Input: part model. Units: mm. Frame: model coordinates. Round coordinates to 2 decimals unless told otherwise and drop trailing zeros. Order: outer loops, then holes, each group sorted by start corner. A loop starts at its lowest first (then second) coordinate and runs counter-clockwise, first axis right, second up. Notation, with made-up numbers: (-17, -28.75) -> (19, -28.75) arc R27 cw to (19, -10.75) -> close; hole circle Ø6 at (39, 28.5). An arc over 180 degrees is marked (long way). Use a Markdown table: item, result.
from build123d import *

# Parameters (mm, degrees)
BASE_DEPTH               = 5
ESQUISSE8_R              = 5
ENL_V_MAT_EXTRU_7_DEPTH  = 10
ESQUISSE4_R              = 11
ESQUISSE4_R_2            = 3.5
ESQUISSE4_RX             = 1.5
ESQUISSE4_RY             = 0.5
ESQUISSE4_W              = 20
ESQUISSE4_H              = 14
ENL_V_MAT_EXTRU_8_DEPTH  = 10
ESQUISSE2_R              = 3
ESQUISSE2_R_2            = 2.5
ENL_V_MAT_EXTRU_9_DEPTH  = 10
ESQUISSE11_R             = 1.5
ENL_V_MAT_EXTRU_11_DEPTH = 5


with BuildPart() as part:
    # Esquisse1 → Base (new body)
    with BuildSketch(Plane.XY):
        Polygon((0, 0), (-175, 0), (-199.748737342, 24.748737342), (-199.748737342, 284.748737342), (-175, 309.497474683), (0, 309.497474683), (24.748737342, 284.748737342), (24.748737342, 24.748737342), align=None)
    extrude(amount=BASE_DEPTH)

    # Esquisse8 → Enlèv. mat.-Extru.7 (cut)
    with BuildSketch(Plane.XY.offset(5)):
        with Locations((-120.5, 286.497474683)):
            Circle(ESQUISSE8_R)
    extrude(amount=-ENL_V_MAT_EXTRU_7_DEPTH, mode=Mode.SUBTRACT)

    # Esquisse4 → Enlèv. mat.-Extru.8 (cut)
    with BuildSketch(Plane.XY.offset(5)):
        with Locations((-87.5, 273.497474683)):
            Circle(ESQUISSE4_R)
        with Locations((-137.5, 274.497474683)):
            Circle(ESQUISSE4_R_2)
        with Locations((-37.5, 274.497474683)):
            Circle(ESQUISSE4_R_2)
        with Locations(Location((-103.5, 286.497474683), (0, 0, -90))):
            Ellipse(ESQUISSE4_RX, ESQUISSE4_RY)
        with Locations(Location((-87.5, 286.497474683), (0, 0, -90))):
            Ellipse(ESQUISSE4_RX, ESQUISSE4_RY)
        with Locations(Location((-71.5, 286.497474683), (0, 0, -90))):
            Ellipse(ESQUISSE4_RX, ESQUISSE4_RY)
        with Locations(Location((-55.5, 286.497474683), (0, 0, -90))):
            Ellipse(ESQUISSE4_RX, ESQUISSE4_RY)
        with Locations((-87.5, 231.748737342)):
            Rectangle(ESQUISSE4_W, ESQUISSE4_H)
    extrude(amount=-ENL_V_MAT_EXTRU_8_DEPTH, mode=Mode.SUBTRACT)

    # Esquisse2 → Enlèv. mat.-Extru.9 (cut)
    with BuildSketch(Plane.XY.offset(5)):
        with Locations((-152.498737342, 23)):
            Circle(ESQUISSE2_R)
        with Locations((-152.498737342, 286.497474683)):
            Circle(ESQUISSE2_R)
        with Locations((-22.501262658, 23)):
            Circle(ESQUISSE2_R)
        with Locations((-22.501262658, 286.497474683)):
            Circle(ESQUISSE2_R)
        with Locations((-137.5, 143.748737342)):
            Circle(ESQUISSE2_R_2)
        with Locations((-126.5, 204.748737342)):
            Circle(ESQUISSE2_R_2)
        with Locations((-37.5, 143.748737342)):
            Circle(ESQUISSE2_R_2)
        with Locations((-48.5, 204.748737342)):
            Circle(ESQUISSE2_R_2)
    extrude(amount=-ENL_V_MAT_EXTRU_9_DEPTH, mode=Mode.SUBTRACT)

    # Esquisse11 → Enlèv. mat.-Extru.11 (cut)
    with BuildSketch(Plane.XY.offset(5)):
        with Locations((-170.614939475, 118.152371839)):
            Circle(ESQUISSE11_R)
        with Locations((-128.614939475, 61.152371839)):
            Circle(ESQUISSE11_R)
        Polygon((-189.748737342, -12.261016229), (-189.748737342, 134.748737342), (-189.748737342, 326.523808624), (-199.748737342, 326.523808624), (-199.748737342, -12.261016229), align=None)
    extrude(amount=-ENL_V_MAT_EXTRU_11_DEPTH, mode=Mode.SUBTRACT)


solid = part.part
1) Pull-direction query (X, two-part tool) for faces 1 (the flat face through (13, 13, 2)), 2 (the flat face through (-81, 157, 5)), 3 (the flat face through (-182, 7, 2)), 4 (the cylindrical face through (-89.88, 262.76, 2.54)); classes: +X half, -X half, draft (parallel to the pull), parting line (faces both ways), or undercut.
Results found:
| item | result |
|---|---|
| face 1 | +X half |
| face 2 | draft |
| face 3 | -X half |
| face 4 | undercut |
2) Cut plane C-C on x = 10. Return loops of the section in (y, z).
Results found:
| item | result |
|---|---|
| outline | (10, 0) -> (299.5, 0) -> (299.5, 5) -> (10, 5) -> close |
3) Pin query (flat end, axial travel): pin 1 Ø5 at (x, y) = (-22.5, 286.5) entering from +Z; pin 2 Ø8 at (x, y) = (-152.5, 23) entering from -Z. Return the tip coordinate at first contact, or that it passes through.
Results found:
| item | result |
|---|---|
| pin 1 | passes through |
| pin 2 | stops at z = 0 |
4) Line query: L1, parallel to Y at x = -137.5, z = 2.65; L2, parallel to Y at x = -48.5, z = 3.9; L3, parallel to Y at x = -78, z = 1.5. Output: solid intervals per line, ascending. Write a range as [from, to].
Results found:
| item | result |
|---|---|
| L1 | y = [0, 141.25], [146.25, 271], [278, 309.5] |
| L2 | y = [0, 202.25], [207.25, 309.5] |
| L3 | y = [0, 224.75], [238.75, 267.95], [279.04, 309.5] |
5) Cut plane B-B on z = 1.5. Count the separate pieces of the cut face and the enclosed holes in it, and give its area (3 significant figures).
Results found:
| item | result |
|---|---|
| separate pieces | 1 |
| enclosed holes | 19 |
| area | 64,500 mm² |
6) Cut plane A-A on x = -120.5. Return loops of the section in (y, z).
Results found:
| item | result |
|---|---|
| outline | (0, 0) -> (281.5, 0) -> (281.5, 5) -> (0, 5) -> close; (291.5, 0) -> (309.5, 0) -> (309.5, 5) -> (291.5, 5) -> close |
